Print and shaded views of the part. All mm, measured from the part's lowest x, y and z. A direction names the side the tool comes from. Round coordinates to 2 decimals unless told otherwise and drop trailing zeros. Order: outer loops, then holes, each group sorted by start corner. A loop starts at its lowest first (then second) coordinate and runs counter-clockwise, first axis right, second up. Notation, with made-up numbers: (-16, 67) - (34, 67) arc R26 cw to (34, 88) - close; hole circle Ø10 at (49, 0). An arc over 180 degrees is marked (long way). Return JSON: item names as keys, results as strings. Group by question number.
Item 1: Drop flat-ended pins along their axis: pin 1 (6 mm diameter, centred on x = 135.5, y = 135, fed in from -Z); pin 2 (1 mm diameter, centred on y = 234.5, z = 202, fed in from +X); pin 3 (10 mm diameter, centred on x = 347.5, y = 218.5, fed in from +Z); pin 4 (1.5 mm diameter, centred on x = 323.5, z = 439, fed in from -Y). Give the stop position or say it passes through.
Item 2: Tool access for the marked faces 1 and 2: list every direction of +Z, -Z, +X, -X, +Y, -Y with a clear straight run to the whole face (end or side of a thin tool).
Item 3: Saw through at B-B on x = 311.5. List the corners of the cut face in (y, z), and give its area (4 significant figures).
Item 4: Saw through at A-A on z = 410. List the corners of the cut face in (x, y).
Item 5: Probe probe 1 along Z at (x, y) = (232, 162); probe 2 along Y at (x, z) = (199.5, 212.5); probe 3 along X at (y, z) = (148.5, 401). List the from-to ranges inside material, lowest first.
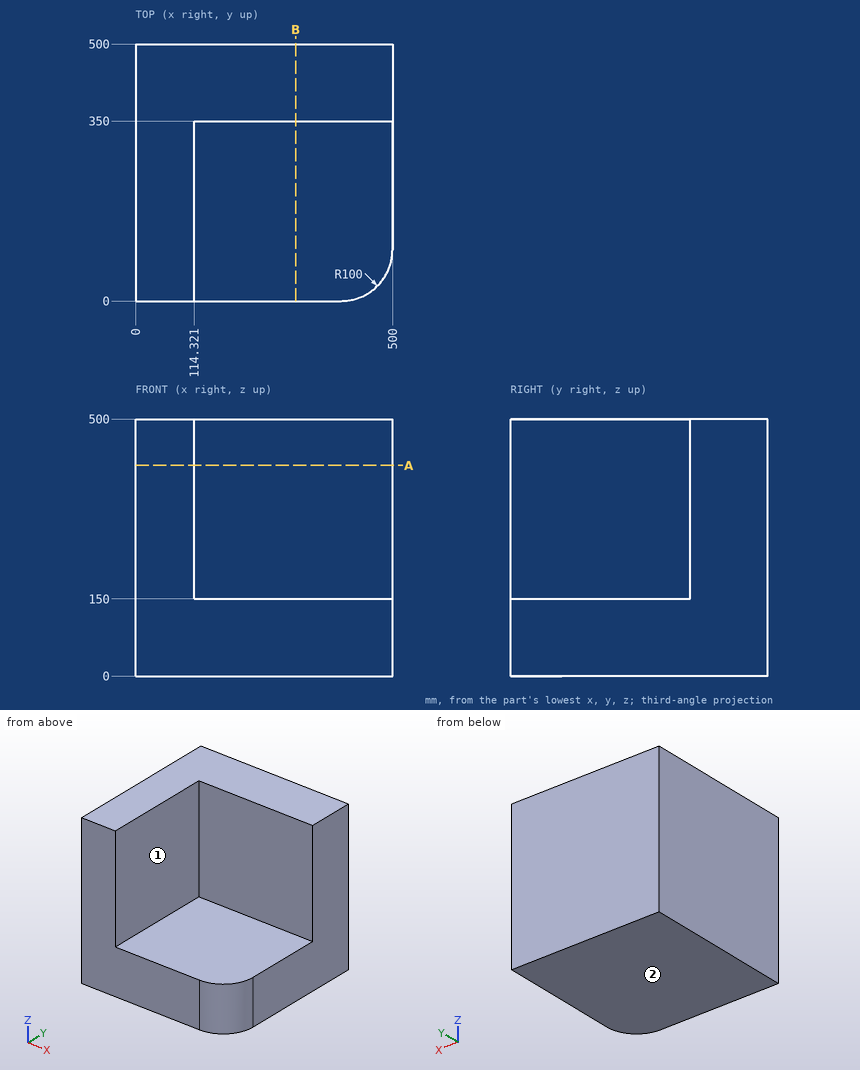
Filled in:
{
 "1": {"pin 1": "stops at z = 0", "pin 2": "stops at x = 114.32", "pin 3": "stops at z = 150", "pin 4": "stops at y = 350"},
 "2": {"face 1": "+Z, +X, -Y", "face 2": "-Z, +X, -X, +Y, -Y"},
 "3": {"outline": "(0, 0) - (500, 0) - (500, 500) - (350, 500) - (350, 150) - (0, 150) - close", "area": "127,500 mm^2"},
 "4": {"outline": "(0, 0) - (114.32, 0) - (114.32, 350) - (500, 350) - (500, 500) - (0, 500) - close"},
 "5": {"probe 1": "z = 0 to 150", "probe 2": "y = 350 to 500", "probe 3": "x = 0 to 114.32"}
}
